The model under review builds one solid part; all positions refer to its coordinate system, in mm. Give positions to 0.01 mm unless a question says otherwise; leave off trailing zeros. Loops run counter-clockwise (first coordinate to the right, second up) from the corner with the lowest first, then second, coordinate; pieces in that order, holes last. Notation, with made-up numbers: (71.25, 10) - (124.25, 10) arc R24 cw to (124.25, 49) - close; hole circle Ø6 at (38.25, 66.5). An arc over 180 degrees is marked (long way). Answer as a JSON object with one key per item and string values.
from build123d import *

# Parameters (mm, degrees)
SZKIC1_R                    = 27.245803964
SZKIC1_R_2                  = 27.636152319
SZKIC1_R_3                  = 50.5
DODANIE_WYCI_GNI_CIE1_DEPTH = 20


with BuildPart() as part:
    # Szkic1 → Dodanie-wyciągnięcie1 (new body)
    with BuildSketch(Plane.XY):
        with BuildLine():
            ThreePointArc((-120.760869565, 74.880102652), (-103.94901291, 77.556678408), (-89.772727273, 86.981937424))
            ThreePointArc((-89.772727273, 86.981937424), (0, 125), (89.772727273, 86.981937424))
            ThreePointArc((89.772727273, 86.981937424), (103.94901291, 77.556678408), (120.760869565, 74.880102652))
            ThreePointArc((120.760869565, 74.880102652), (200, 0), (120.760869565, -74.880102652))
            ThreePointArc((120.760869565, -74.880102652), (103.94901291, -77.556678408), (89.772727273, -86.981937424))
            ThreePointArc((89.772727273, -86.981937424), (0, -125), (-89.772727273, -86.981937424))
            ThreePointArc((-89.772727273, -86.981937424), (-103.94901291, -77.556678408), (-120.760869565, -74.880102652))
            ThreePointArc((-120.760869565, -74.880102652), (-200, 0), (-120.760869565, 74.880102652))
        make_face()
        with Locations((125, 0)):
            Circle(SZKIC1_R, mode=Mode.SUBTRACT)
        with Locations((-125, 0)):
            Circle(SZKIC1_R_2, mode=Mode.SUBTRACT)
        Circle(SZKIC1_R_3, mode=Mode.SUBTRACT)
    extrude(amount=DODANIE_WYCI_GNI_CIE1_DEPTH)


solid = part.part
Q1. Consider section B-B, the plane y = 0. State the section outline as (x, z) points, plus the area to 3 significant figures.
Results:
{"outline": "(-200, 0) - (-152.64, 0) - (-152.64, 20) - (-200, 20) - close; (-97.36, 0) - (-50.5, 0) - (-50.5, 20) - (-97.36, 20) - close; (50.5, 0) - (97.75, 0) - (97.75, 20) - (50.5, 20) - close; (152.25, 0) - (200, 0) - (200, 20) - (152.25, 20) - close", "area": "3,780 mm^2"}
Q2. Consider section D-D, the plane x = 125. State the section outline as (y, z) points.
Results:
{"outline": "(-75, 0) - (-27.25, 0) - (-27.25, 20) - (-75, 20) - close; (27.25, 0) - (75, 0) - (75, 20) - (27.25, 20) - close"}
Q3. To check wall thickness, follow probe 1 along X at (y, z) = (4.5, 18.5); probe 2 along Y at (x, z) = (125, 10); probe 3 along Y at (x, z) = (-44, 9.75). State the ranges of each line that lie inside material, in increasing order. Write a range as [from, to].
Results:
{"probe 1": "x = [-199.86, -152.27], [-97.73, -50.3], [50.3, 98.13], [151.87, 199.86]", "probe 2": "y = [-75, -27.25], [27.25, 75]", "probe 3": "y = [-117, -24.78], [24.78, 117]"}
Q4. Consider section A-A, the plane x = -125. State the section outline as (y, z) points, plus the area to 3 significant figures.
Results:
{"outline": "(-75, 0) - (-27.64, 0) - (-27.64, 20) - (-75, 20) - close; (27.64, 0) - (75, 0) - (75, 20) - (27.64, 20) - close", "area": "1,890 mm^2"}
Q5. The part is to be moulded in two halves that separate along Y. For faces 1 (the face through (97.78, 1.2, 9.86)), 2 (the face through (-103.726, -77.645, 9.86)), 3 (the face through (-104.17, 77.47, 9.86)), 4 (the face through (199.98, 1.71, 9.86)), say which applies: +Y half, -Y half, draft (parallel to the pull), parting line (faces both ways), or undercut.
Results:
{"face 1": "undercut", "face 2": "-Y half", "face 3": "+Y half", "face 4": "parting line"}
Q6. Consider section C-C, the plane z = 3.75. State the section outline as (x, y) points, plus the area to 3 significant figures.
Results:
{"outline": "(-120.76, -74.88) arc R40 cw to (-89.77, -86.98) arc R125 ccw to (89.77, -86.98) arc R40 cw to (120.76, -74.88) arc R75 ccw (long way) to (120.76, 74.88) arc R40 cw to (89.77, 86.98) arc R125 ccw to (-89.77, 86.98) arc R40 cw to (-120.76, 74.88) arc R75 ccw (long way) to start; hole circle Ø55.27 at (-125, 0); hole circle Ø101 at (0, 0); hole circle Ø54.49 at (125, 0)", "area": "56,600 mm^2"}
Q7. Clearance check with flat-ended pins moving along their axes: pin 1 Ø6 at (y, z) = (84, 6) entering from -X; pin 2 Ø12 at (y, z) = (68, 6.5) entering from +X; pin 3 Ø1 at (y, z) = (-86, 17.5) entering from +X. State where each tip first meets the part, or that it passes through.
Results:
{"pin 1": "stops at x = -97.13", "pin 2": "stops at x = 167.2", "pin 3": "stops at x = 91.29"}
